```python
from build123d import *

# Parameters (mm, degrees)
SKETCH1_R                 = 13.95
BOSS_EXTRUDE1_DEPTH       = 25.7
CHAMFER1_SIZE             = 3
CHAMFER1_SIZE2            = 5
SKETCH2_R                 = 4
BOSS_EXTRUDE2_DEPTH       = 14
M3X0_5_TAPPED_HOLE1_D     = 2.5
M3X0_5_TAPPED_HOLE1_DEPTH = 7.5
M3X0_5_TAPPED_HOLE1_TIP   = 0.751075774
FILLET1_R                 = 3
SKETCH5_R                 = 3
BOSS_EXTRUDE3_DEPTH       = 2.5


with BuildPart() as part:
    # Sketch1 → Boss-Extrude1 (new body)
    with BuildSketch(Plane(origin=(0, 0, 0), x_dir=(1, 0, 0), z_dir=(0, 1, 0))):
        Circle(SKETCH1_R)
    extrude(amount=BOSS_EXTRUDE1_DEPTH)

    # Chamfer1
    chamfer1_edges = [part.edges().sort_by_distance(p)[0] for p in [
        (-13.95, 25.7, 0),
    ]]
    chamfer1_side = [part.faces().sort_by_distance(p)[0] for p in [
        (-13.95, 12.85, 0),
    ]]
    chamfer(chamfer1_edges, length=CHAMFER1_SIZE, length2=CHAMFER1_SIZE2, reference=chamfer1_side[0])

    # Sketch2 → Boss-Extrude2 (add)
    with BuildSketch(Plane(origin=(0, 25.7, 0), x_dir=(1, 0, 0), z_dir=(0, 1, 0))):
        Circle(SKETCH2_R)
    extrude(amount=BOSS_EXTRUDE2_DEPTH)

    # M3x0.5 Tapped Hole1
    with Locations(Plane(origin=(0, 0, 0), x_dir=(-1, 0, 0), z_dir=(0, -1, 0))):
        with Locations((0, 8), (0, -8), (-9.5, 0), (9.5, 0)):
            Hole(M3X0_5_TAPPED_HOLE1_D / 2, depth=M3X0_5_TAPPED_HOLE1_DEPTH)
            with Locations((0, 0, -(M3X0_5_TAPPED_HOLE1_DEPTH + M3X0_5_TAPPED_HOLE1_TIP / 2))):  # 118° drill point
                Cone(0, M3X0_5_TAPPED_HOLE1_D / 2, M3X0_5_TAPPED_HOLE1_TIP, mode=Mode.SUBTRACT)

    # Fillet1
    fillet1_edges = [part.edges().sort_by_distance(p)[0] for p in [
        (-13.95, 0, 0),
    ]]
    fillet(fillet1_edges, radius=FILLET1_R)

    # Sketch5 → Boss-Extrude3 (add)
    with BuildSketch(Plane.XZ):
        Circle(SKETCH5_R)
    extrude(amount=BOSS_EXTRUDE3_DEPTH)


solid = part.part
```
The listing builds one solid part. Answer for the finished solid, in the listing's coordinates (mm). A direction names the side the tool comes from. Give positions to 0.01 mm unless a question says otherwise; leave off trailing zeros. Loops run counter-clockwise (first coordinate to the right, second up) from the corner with the lowest first, then second, coordinate; pieces in that order, holes last. Notation, with made-up numbers: (69, 12) - (104, 12) arc R28 ccw to (104, 49) - close; hole circle Ø9 at (-29.5, -11). An arc over 180 degrees is marked (long way). Return JSON: item names as keys, results as strings. Group by question number.
1. Determine the mould class of faces 1 (the cylindrical face through (-0.27, 3.8, 9.22)), 2 (the cylindrical face through (-3.02, 12.71, 13.62)), 3 (the flat face through (2.3, 0, 2.3)) for opening direction Z: pulls with the +Z half, pulls with the -Z half, needs draft (parallel to the pull), parting line crosses it, or undercut.
2. Find section B-B (y = 14). Write down the section's boundary in (x, z), then the cut area to 3 significant figures.
3. Given pin 1 Ø2 at (x, z) = (9.5, 0) entering from -Y; pin 2 Ø6 at (x, y) = (-5, 16) entering from -Z; pin 3 Ø5 at (x, z) = (-9.5, -1.5) entering from +Y, each flat-ended and moving along its own axis, determine where each tip first touches the part or whether it passes through.
4. Straight lines are drawn through the part: line 1 (Z direction, x = 0, y = 4.5); line 2 (Z direction, x = -9.5, y = 3.25); line 3 (Y direction, x = 4.5, z = 1.75). For each, find the intervals that lie inside material, in ascending order. Write a range as [from, to].
5. Find section A-A (y = 4). Write down the section's boundary in (x, z), then the cut area to 3 significant figures.
6. Which of the six approach directions +Z, -Z, +X, -X, +Y, -Y give full straight-line access (tool end or side, diameter ignored) to faces 4 (the flat face through (0, -2.5, 0)), 5 (the cylindrical face through (-10.75, 3.8, -0.05)), 6 (the cylindrical face through (-0.867, 32.602, 3.905))?
Verdict:
{
 "1": {"face 1": "undercut", "face 2": "parting line crosses it", "face 3": "needs draft"},
 "2": {"outline": "circle Ø27.9 at (0, 0)", "area": "611 mm^2"},
 "3": {"pin 1": "stops at y = 7.65", "pin 2": "stops at z = -13.81", "pin 3": "stops at y = 25.7"},
 "4": {"line 1": "z = [-13.95, -9.25], [-6.75, 6.75], [9.25, 13.95]", "line 2": "z = [-10.22, -1.25], [1.25, 10.22]", "line 3": "y = [0, 25.7]"},
 "5": {"outline": "circle Ø27.9 at (0, 0); hole circle Ø2.5 at (-9.5, 0); hole circle Ø2.5 at (0, -8); hole circle Ø2.5 at (0, 8); hole circle Ø2.5 at (9.5, 0)", "area": "592 mm^2"},
 "6": {"face 4": "+Z, -Z, +X, -X, -Y", "face 5": "-Y", "face 6": "+Y"}
}
